Autodesk Inventor part; units mm, degrees
ref_plane "YZ Plane" through (0, 0, 0) normal (1, 0, 0) x (0, 1, 0)
ref_plane "XZ Plane" through (0, 0, 0) normal (0, 1, 0) x (-1, 0, 0)
ref_plane "XY Plane" through (0, 0, 0) normal (0, 0, 1) x (1, 0, 0)
sketch "Sketch1" plane through (0, 0, 0) normal (0, 1, 0) x (-1, 0, 0)
  line L0 (0, 0) -> (173.228, 0)
  line L1 (173.228, 0) -> (173.228, -330.2)
  line L2 (173.228, -330.2) -> (0, -330.2)
  line L3 (0, -330.2) -> (0, 0)
  dimension "d0" = 173.228
  dimension "d1" = 330.2
extrude "Extrusion1" add sketch "Sketch1" along normal blind 251.46
fillet "Fillet1" radius 3.175 12 edges at (0, 251.46, -165.1) (-86.614, 251.46, 0) (0, 125.73, 0) (-173.228, 251.46, -165.1) (-86.614, 251.46, -330.2) (0, 125.73, -330.2) (-173.228, 125.73, 0) (-86.614, 0, 0) (0, 0, -165.1) (-173.228, 0, -165.1) (-86.614, 0, -330.2) (-173.228, 125.73, -330.2)
sketch "Sketch2" plane through (0, 251.46, 0) normal (0, 1, 0) x (1, 0, 0)
  circle A0 centre (-86.614, 63.5) radius 3.175
  circle A1 centre (-86.614, 266.7) radius 3.175
  line L0 (0, 3.175) -> (0, 327.025)
  line L1 (-173.228, 327.025) -> (-173.228, 3.175)
  line L2 (-3.175, 330.2) -> (-170.053, 330.2)
  line L3 (-170.053, 0) -> (-3.175, 0)
  point P0 (0, 0)
  dimension "d5" = 6.35
  dimension "d6" = 6.35
  dimension "d9" = 86.614
  dimension "d10" = 86.614
  dimension "d11" = 86.614
  dimension "d12" = 63.5
  dimension "d13" = 63.5
extrude "Extrusion2" add sketch "Sketch2" along normal blind 19.05
fillet "Fillet2" radius 3.175 2 edges at (-89.789, 270.51, -63.5) (-89.789, 270.51, -266.7)
equation "\"d10\" = d11"
properties part number "Deep Cycle Battery"
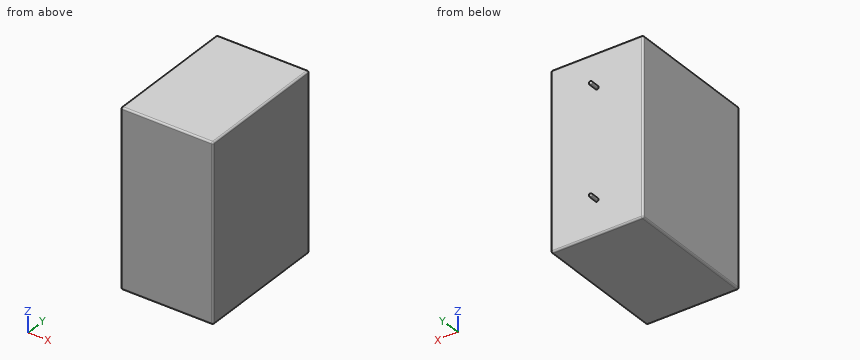
CAD build for the part. Positions are in the model's coordinates, mm. Round coordinates to 2 decimals unless told otherwise and drop trailing zeros. Order: outer loops, then holes, each group sorted by start corner. A loop starts at its lowest first (then second) coordinate and runs counter-clockwise, first axis right, second up. Notation, with made-up numbers: (20, 63.5) - (32, 63.5) arc R21 ccw to (32, 76.5) - close; hole circle Ø6 at (-30, 27). An arc over 180 degrees is marked (long way). Return JSON: item names as keys, results as strings.
(1) Pin check, flat tips, straight feed: pin 1 Ø6 at (y, z) = (88, -245.5) entering from +X; pin 2 Ø4 at (x, z) = (-84.5, -95) entering from +Y. Stop position of each tip, or through.
Answer key:
{"pin 1": "stops at x = 0", "pin 2": "stops at y = 251.46"}
(2) Cut at B-B (z = -118). Give the cut face in (x, y) (3 decimals).
Answer key:
{"outline": "(-173.228, 3.175) arc R3.175 ccw to (-170.053, 0) - (-3.175, 0) arc R3.175 ccw to (0, 3.175) - (0, 248.285) arc R3.175 ccw to (-3.175, 251.46) - (-170.053, 251.46) arc R3.175 ccw to (-173.228, 248.285) - close"}
(3) Cut at A-A (x = -157). Give the cut face in (y, z) (3 decimals), then the cut area to 3 significant figures.
Answer key:
{"outline": "(0, -327.025) arc R3.175 ccw to (3.175, -330.2) - (248.285, -330.2) arc R3.175 ccw to (251.46, -327.025) - (251.46, -3.175) arc R3.175 ccw to (248.285, 0) - (3.175, 0) arc R3.175 ccw to (0, -3.175) - close", "area": "83,000 mm^2"}
(4) Wall check: probe 1 along Y at (x, z) = (-79, -278). Give the ranges that are in metal, low to high. Write a range as from..to.
Answer key:
{"probe 1": "y = 0..251.46"}
